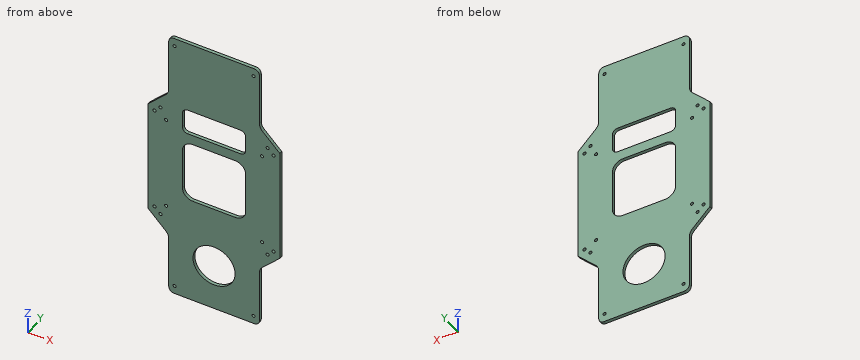
from build123d import *

# Parameters (mm, degrees)
SKETCH_1_R          = 1.5
EXTRUDE_1_DEPTH     = 3
CHAMFER_1_SIZE      = 7
SKETCH_3_W          = 60
SKETCH_3_H          = 60
SKETCH_3_R          = 1.5
SKETCH_3_R_2        = 20
SKETCH_3_H_2        = 10
SKETCH_3_H_3        = 5
CUT_EXTRUDE_1_DEPTH = 3
FILLET_3_R          = 10
FILLET_4_R          = 5
FILLET_5_R          = 5
CHAMFER_2_SIZE      = 12.5
FILLET_6_R          = 10


with BuildPart() as part:
    # 草图1 → 凸台-拉伸1 (new body)
    with BuildSketch(Plane(origin=(0, 0, 0), x_dir=(1, 0, 0), z_dir=(0, 1, 0))):
        Polygon((-62.5, 62.5), (-62.5, -62.5), (-43, -62.5), (-43, -135), (43, -135), (43, -62.5), (62.5, -62.5), (62.5, 62.5), (43, 62.5), (43, 135), (-43, 135), (-43, 62.5), align=None)
        with Locations(Location((-56.5, -50.843145751, 0), (0, 0, 270))):
            Circle(SKETCH_1_R, mode=Mode.SUBTRACT)
        with Locations(Location((-50.843145751, -56.5, 0), (0, 0, 270))):
            Circle(SKETCH_1_R, mode=Mode.SUBTRACT)
        with Locations(Location((50.843145751, -56.5, 0), (0, 0, 270))):
            Circle(SKETCH_1_R, mode=Mode.SUBTRACT)
        with Locations(Location((56.5, -50.843145751, 0), (0, 0, 270))):
            Circle(SKETCH_1_R, mode=Mode.SUBTRACT)
        with Locations(Location((-56.5, 50.843145751, 0), (0, 0, 270))):
            Circle(SKETCH_1_R, mode=Mode.SUBTRACT)
        with Locations(Location((-50.843145751, 56.5, 0), (0, 0, 270))):
            Circle(SKETCH_1_R, mode=Mode.SUBTRACT)
        with Locations(Location((50.843145751, 56.5, 0), (0, 0, 270))):
            Circle(SKETCH_1_R, mode=Mode.SUBTRACT)
        with Locations(Location((56.5, 50.843145751, 0), (0, 0, 270))):
            Circle(SKETCH_1_R, mode=Mode.SUBTRACT)
        with Locations(Location((37.5, -127, 0), (0, 0, 270))):
            Circle(SKETCH_1_R, mode=Mode.SUBTRACT)
        with Locations(Location((-37.5, -127, 0), (0, 0, 270))):
            Circle(SKETCH_1_R, mode=Mode.SUBTRACT)
        with Locations(Location((37.5, 127, 0), (0, 0, 270))):
            Circle(SKETCH_1_R, mode=Mode.SUBTRACT)
        with Locations(Location((-37.5, 127, 0), (0, 0, 270))):
            Circle(SKETCH_1_R, mode=Mode.SUBTRACT)
    extrude(amount=EXTRUDE_1_DEPTH)

    # 倒角1
    chamfer_1_edges = [part.edges().sort_by_distance(p)[0] for p in [
        (-62.5, 1.5, 62.5),
        (-62.5, 1.5, -62.5),
        (62.5, 1.5, -62.5),
        (62.5, 1.5, 62.5),
    ]]
    chamfer(chamfer_1_edges, length=CHAMFER_1_SIZE)

    # 草图3 → 切除-拉伸1 (cut)
    with BuildSketch(Plane(origin=(0, 3, 0), x_dir=(1, 0, 0), z_dir=(0, 1, 0))):
        Rectangle(SKETCH_3_W, SKETCH_3_H)
        with Locations(Location((-45.5, 45.5, 0), (0, 0, 270))):
            Circle(SKETCH_3_R)
        with Locations(Location((45.5, 45.5, 0), (0, 0, 270))):
            Circle(SKETCH_3_R)
        with Locations(Location((45.5, -45.5, 0), (0, 0, 270))):
            Circle(SKETCH_3_R)
        with Locations(Location((-45.5, -45.5, 0), (0, 0, 270))):
            Circle(SKETCH_3_R)
        with Locations(Location((0, 90, 0), (0, 0, 270))):
            Circle(SKETCH_3_R_2)
        with Locations((0, -44.5)):
            Rectangle(SKETCH_3_W, SKETCH_3_H_2)
        with Locations((0, -54.5)):
            Rectangle(SKETCH_3_W, SKETCH_3_H_2)
        with Locations((0, -62)):
            Rectangle(SKETCH_3_W, SKETCH_3_H_3)
    extrude(amount=-CUT_EXTRUDE_1_DEPTH, mode=Mode.SUBTRACT)

    # 圆角3
    fillet_3_edges = [part.edges().sort_by_distance(p)[0] for p in [
        (30, 1.5, 30),
        (-30, 1.5, 30),
        (-30, 1.5, -30),
        (30, 1.5, -30),
    ]]
    fillet(fillet_3_edges, radius=FILLET_3_R)

    # 圆角4
    fillet_4_edges = [part.edges().sort_by_distance(p)[0] for p in [
        (-43, 1.5, -135),
        (43, 1.5, -135),
        (43, 1.5, 135),
        (-43, 1.5, 135),
    ]]
    fillet(fillet_4_edges, radius=FILLET_4_R)

    # 圆角5
    fillet_5_edges = [part.edges().sort_by_distance(p)[0] for p in [
        (30, 1.5, 39.5),
        (30, 1.5, 64.5),
        (-30, 1.5, 64.5),
        (-30, 1.5, 39.5),
    ]]
    fillet(fillet_5_edges, radius=FILLET_5_R)

    # 倒角2
    chamfer_2_edges = [part.edges().sort_by_distance(p)[0] for p in [
        (43, 1.5, -62.5),
        (-43, 1.5, -62.5),
        (43, 1.5, 62.5),
        (-43, 1.5, 62.5),
    ]]
    chamfer(chamfer_2_edges, length=CHAMFER_2_SIZE - 0.0001)  # a hair under: the kernel refuses the full size

    # 圆角6
    fillet_6_edges = [part.edges().sort_by_distance(p)[0] for p in [
        (43, 1.5, -74.9999),
        (-43, 1.5, -74.9999),
        (43, 1.5, 74.9999),
        (-43, 1.5, 74.9999),
    ]]
    fillet(fillet_6_edges, radius=FILLET_6_R)


solid = part.part
The listing builds one solid part. Answer for the finished solid, in the listing's coordinates (mm). Give positions to 0.01 mm unless a question says otherwise; leave off trailing zeros. Write each loop counter-clockwise with the first axis right and the second up, starting at its lowest first coordinate (ties: lowest second). Pieces come first, ordered by that corner, then holes. Notation, with made-up numbers: (-14.5, 66.25) - (-2.5, 66.25) arc R17 cw to (-2.5, 80.25) - close; hole circle Ø2 at (88, -26.75). An arc over 180 degrees is marked (long way). One line per question, with ' | ' between items. Start each with the question number.
1. Straight lines are drawn through the part: line 1 (X direction, y = 2.25, z = 45.5); line 2 (X direction, y = 2.25, z = 127); line 3 (X direction, y = 1.1, z = 14). For each, find the intervals that lie inside material, in ascending order.
2. Section D-D, the plane y = 2.4 is taken. Count the separate pieces of the cut face and the enclosed holes in it, then the cut area to 3 significant figures.
3. Given P1, Ø3, axis at x = -32, z = 57, coming from the -Y side; P2, Ø2.5, axis at x = -37.5, z = -127, coming from the -Y side; P3, Ø1.5, axis at y = 2, z = 109.5, coming from the +X side, each flat-ended and moving along its own axis, determine where each tip first touches the part or whether it passes through.
4. Section B-B, the plane x = 12 is taken. Determine the outline of the cut face in (y, z).
5. Section C-C, the plane z = -90 is taken. Determine the outline of the cut face in (x, y), then the cut area to 3 significant figures.
6. Section A-A, the plane z = 17 is taken. Determine the outline of the cut face in (x, y), then the cut area to 3 significant figures.
Result:
1) line 1: x = -62.5 to -47, -44 to -30, 30 to 44, 47 to 62.5 | line 2: x = -43 to -39, -36 to 36, 39 to 43 | line 3: x = -62.5 to -30, 30 to 62.5
2) separate pieces: 1 | enclosed holes: 19 | area: 21,900 mm2
3) P1: stops at y = 0 | P2: passes through | P3: stops at x = 43
4) outline: (0, -135) - (3, -135) - (3, -106) - (0, -106) - close; (0, -74) - (3, -74) - (3, -30) - (0, -30) - close; (0, 30) - (3, 30) - (3, 39.5) - (0, 39.5) - close; (0, 64.5) - (3, 64.5) - (3, 135) - (0, 135) - close
5) outline: (-43, 0) - (-20, 0) - (-20, 3) - (-43, 3) - close; (20, 0) - (43, 0) - (43, 3) - (20, 3) - close | area: 138 mm2
6) outline: (-62.5, 0) - (-30, 0) - (-30, 3) - (-62.5, 3) - close; (30, 0) - (62.5, 0) - (62.5, 3) - (30, 3) - close | area: 195 mm2
